Check sheet for the modelled part. Datum: model origin and axes. Units: mm. Coordinates: 2 decimals unless noted, no trailing zeros. Loops run counter-clockwise (first coordinate to the right, second up) from the corner with the lowest first, then second, coordinate; pieces in that order, holes last. Notation, with made-up numbers: (5, 70.25) -> (34, 70.25) arc R23 cw to (34, 99.25) -> close; hole circle Ø8 at (6, 77.5). An arc over 180 degrees is marked (long way). Use CSV: the item, a comma, the result in double quotes. Start each with the question number.
1. Sectioned sample at C-C, the plane z = 50.5. Record the cut outline in (x, y), and give its area (3 significant figures).
2. Thickness scan on L1, parallel to Y at x = -68, z = 2; L2, parallel to Z at x = 14, y = 36; L3, parallel to Y at x = -32, z = 23.5. Record the ranges inside material, lowest first.
3. Gauge pin test, flat ends, axial feed: pin 1 (5 mm diameter, centred on x = 58, z = -41, fed in from -Y); pin 2 (8 mm diameter, centred on x = 14.5, z = 11, fed in from +Y); pin 3 (4 mm diameter, centred on x = 57.5, y = 21, fed in from +Z). Record the tip position at first contact, or that the pin passes through.
4. Sectioned sample at B-B, the plane y = 34.5. Record the cut outline in (x, z).
```python
from build123d import *

# Parameters (mm, degrees)
F1_W     = 170
F1_H     = 150
F2_DEPTH = 10
F3_SIZE  = 9.99999


# Not quite as in the source:
# - a fillet or chamfer is up to 0.001 mm smaller than in the source, because OpenCascade refuses the exact size


with BuildPart() as f2:
    # F1 (on face) → F2 (new body)
    with BuildSketch(Plane(origin=(0, 0, 0), x_dir=(-1, 0, 0), z_dir=(0, 0.7071067812, 0.7071067812))):
        Rectangle(F1_W, F1_H)
    extrude(amount=F2_DEPTH)

    # F3 (size 10 in the source; OpenCascade refuses exactly that, so slightly less here)
    f3_edges = [f2.edges().sort_by_distance(p)[0] for p in [
        (0, -53.033009, 53.033009),
    ]]
    chamfer(f3_edges, length=F3_SIZE)


solid = f2.part
```
Completed:
1,outline,"(-85, -45.96) -> (85, -45.96) -> (85, -36.36) -> (-85, -36.36) -> close"
1,area,"1,630 mm²"
2,L1,"-2 to 12.14"
2,L2,"-36 to -21.86"
2,L3,"-23.5 to -9.36"
3,pin 1,"y = 38.5"
3,pin 2,"y = 7.14"
3,pin 3,"z = -4.86"
4,outline,"(-85, -34.5) -> (85, -34.5) -> (85, -20.36) -> (-85, -20.36) -> close"
